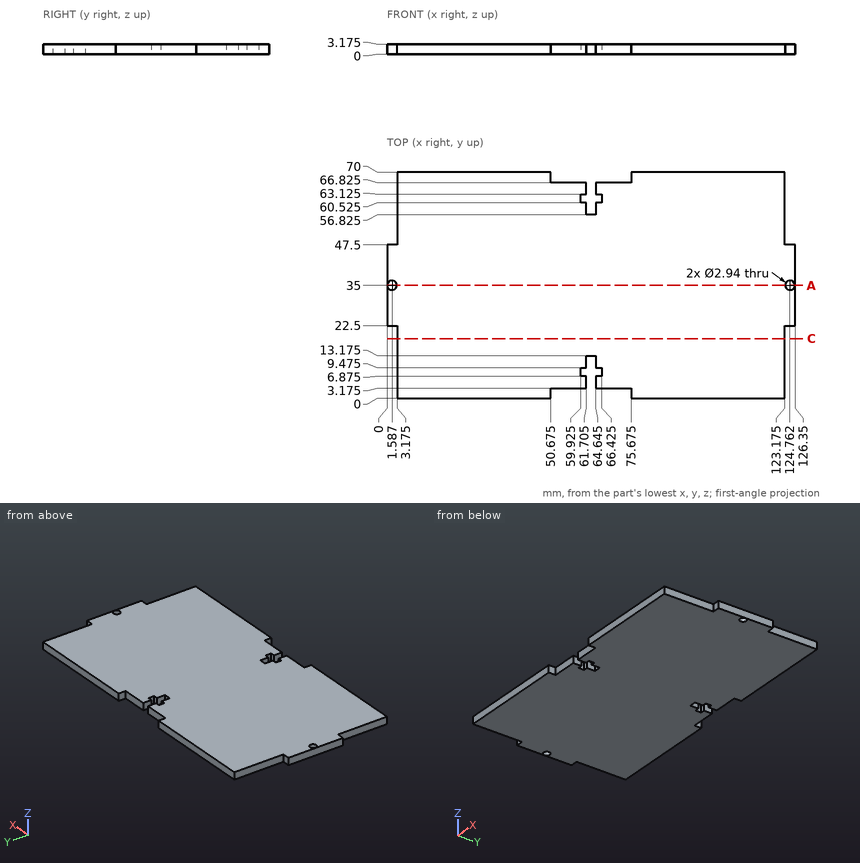
Design review of the part shown in the three views and the two pictorial views. Dimensions are in mm from the part's minimum x, y and z. Round coordinates to 2 decimals unless told otherwise and drop trailing zeros. Write each loop counter-clockwise with the first axis right and the second up, starting at its lowest first coordinate (ties: lowest second). Pieces come first, ordered by that corner, then holes. Notation, with made-up numbers: M 42,-3.75 L 63,-3.75 A27 cw 63,23.25 Z; hole C -40,47.5 d11. An arc over 180 degrees is marked long. One line per item, written item: value. Start each with the question number.
1. Clearance check with flat-ended pins moving along their axes: P1, Ø1.5, axis at x = 62.5, z = 2, coming from the +Y side (1 decimal); P2, Ø0.8, axis at y = 8, z = 1.5, coming from the +X side (1 decimal); P3, Ø1, axis at x = 72, z = 2, coming from the +Y side (1 decimal). State where each tip first meets the part, or that it passes through.
2. Take a section at C-C on y = 18.5. State the section outline as (x, z) points (1 decimal).
3. Take a section at A-A on y = 35. State how many separate pieces and enclosed holes the cut face has.
4. To check wall thickness, follow probe 1 along X at (y, z) = (11, 2.6) (1 decimal); probe 2 along X at (y, z) = (51, 1.4) (1 decimal); probe 3 along Y at (x, z) = (56, 3.05) (1 decimal). State the ranges of each line that lie inside material, in increasing order. Write a range as from..to.
Computed:
1. P1: stops at y = 56.8
1. P2: stops at x = 123.2
1. P3: stops at y = 66.8
2. outline: M 3.2,0 L 123.2,0 L 123.2,3.2 L 3.2,3.2 Z
3. separate pieces: 3
3. enclosed holes: 0
4. probe 1: x = 3.2..61.7, 64.6..123.2
4. probe 2: x = 3.2..123.2
4. probe 3: y = 3.2..66.8
